Can you work these out from the model? Positions are in its coordinate system, mm. Face numbers are marked on the shaded views. A direction names the side the tool comes from. Give positions to 0.01 mm unless a question says otherwise; leave off trailing zeros. Loops run counter-clockwise (first coordinate to the right, second up) from the corner with the lowest first, then second, coordinate; pieces in that order, holes last. Notation, with made-up numbers: M -15,87.25 L 32,87.25 A38 ccw 32,126.25 Z; hole C -33,-28.75 d4. An arc over 180 degrees is marked long. Answer as a JSON object with one key per item and string values.
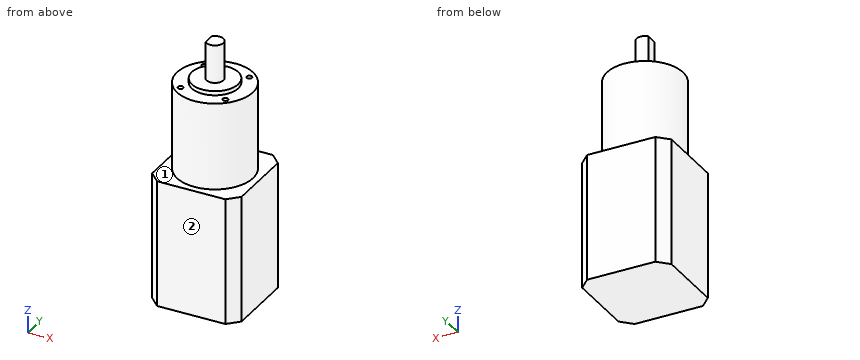
```python
from build123d import *

# Parameters (mm, degrees)
EXTRUDE_1_DEPTH        = 60
SKETCH_2_R             = 18
EXTRUDE_2_DEPTH        = 41.3
SKETCH_3_R             = 11
EXTRUDE_3_DEPTH        = 2
SKETCH_4_R             = 4
EXTRUDE_4_DEPTH        = 18
SKETCH_5_W             = 8.09428643
SKETCH_5_H             = 13.450799509
CUT_EXTRUDE_1_DEPTH    = 15
SKETCH_6_R             = 1
CUT_EXTRUDE_2_DEPTH    = 5
HOLE_WIZARD_M3_1_D     = 2.5
HOLE_WIZARD_M3_1_DEPTH = 7.5
HOLE_WIZARD_M3_1_TIP   = 0.751075774


with BuildPart() as part:
    # 草图1 → 凸台-拉伸1 (new body)
    with BuildSketch(Plane.XY):
        Polygon((-21.15, 16.15), (-16.15, 21.15), (16.15, 21.15), (21.15, 16.15), (21.15, -16.15), (16.15, -21.15), (-16.15, -21.15), (-21.15, -16.15), align=None)
    extrude(amount=EXTRUDE_1_DEPTH)

    # 草图2 → 凸台-拉伸2 (add)
    with BuildSketch(Plane.XY.offset(60)):
        Circle(SKETCH_2_R)
    extrude(amount=EXTRUDE_2_DEPTH)

    # 草图3 → 凸台-拉伸3 (add)
    with BuildSketch(Plane.XY.offset(101.3)):
        Circle(SKETCH_3_R)
    extrude(amount=EXTRUDE_3_DEPTH)

    # 草图4 → 凸台-拉伸4 (add)
    with BuildSketch(Plane.XY.offset(103.3)):
        Circle(SKETCH_4_R)
    extrude(amount=EXTRUDE_4_DEPTH)

    # 草图5 → 切除-拉伸1 (cut)
    with BuildSketch(Plane.XY.offset(121.3)):
        with Locations((-7.047143215, -1.347451383)):
            Rectangle(SKETCH_5_W, SKETCH_5_H)
    extrude(amount=-CUT_EXTRUDE_1_DEPTH, mode=Mode.SUBTRACT)

    # 草图6 → 切除-拉伸2 (cut)
    with BuildSketch(Plane.XY.offset(101.3)):
        with Locations((-10.606601718, 10.606601718)):
            Circle(SKETCH_6_R)
        with Locations((10.606601718, 10.606601718)):
            Circle(SKETCH_6_R)
        with Locations((-10.606601718, -10.606601718)):
            Circle(SKETCH_6_R)
        with Locations((10.606601718, -10.606601718)):
            Circle(SKETCH_6_R)
    extrude(amount=-CUT_EXTRUDE_2_DEPTH, mode=Mode.SUBTRACT)

    # M3 螺纹孔1
    with Locations(Plane.XY.offset(101.3)):
        with Locations((-10.606601718, 10.606601718), (10.606601718, 10.606601718), (-10.606601718, -10.606601718), (10.606601718, -10.606601718)):
            Hole(HOLE_WIZARD_M3_1_D / 2, depth=HOLE_WIZARD_M3_1_DEPTH)
            with Locations((0, 0, -(HOLE_WIZARD_M3_1_DEPTH + HOLE_WIZARD_M3_1_TIP / 2))):  # 118° drill point
                Cone(0, HOLE_WIZARD_M3_1_D / 2, HOLE_WIZARD_M3_1_TIP, mode=Mode.SUBTRACT)


solid = part.part
```
1) Suppose I cut it at D-D, the plane y = 14.5. Write out the boundary of the cut face in (x, z).
Answer list:
{"outline": "M -21.15,0 L 21.15,0 L 21.15,60 L 10.67,60 L 10.67,101.3 L -10.67,101.3 L -10.67,60 L -21.15,60 Z"}
2) Will these pins go through, and if not, where does the flat tip stop? pin 1 Ø8 at (y, z) = (-5.5, 67.5) entering from -X; pin 2 Ø21 at (x, y) = (-9, -6) entering from +Z; pin 3 Ø8 at (x, z) = (16, 88.5) entering from +Y; pin 4 Ø3 at (x, z) = (-1, 77.5) entering from +Y.
Answer list:
{"pin 1": "x = -17.94", "pin 2": "z = 121.3", "pin 3": "y = 13.42", "pin 4": "y = 18"}
3) Suppose I cut it at C-C, the plane z = 58.5. Write out the boundary of the cut face in (x, y), and give its area (3 significant figures).
Answer list:
{"outline": "M -21.15,-16.15 L -16.15,-21.15 L 16.15,-21.15 L 21.15,-16.15 L 21.15,16.15 L 16.15,21.15 L -16.15,21.15 L -21.15,16.15 Z", "area": "1,740 mm^2"}
4) For the marked faces 1 and 2, which set-ups out of +Z, -Z, +X, -X, +Y, -Y let a thin tool reach every point of the face, with its end or its side?
Answer list:
{"face 1": "+Z", "face 2": "+Z, -Z, +X, -X, -Y"}
5) Suppose I cut it at B-B, the plane x = 0. Write out the boundary of the cut face in (y, z).
Answer list:
{"outline": "M -21.15,0 L 21.15,0 L 21.15,60 L 18,60 L 18,101.3 L 11,101.3 L 11,103.3 L 4,103.3 L 4,121.3 L -4,121.3 L -4,103.3 L -11,103.3 L -11,101.3 L -18,101.3 L -18,60 L -21.15,60 Z"}
6) Please list where these lines run through material, in increasing order: line 1 along Z through (x, y) = (-4.5, 1.5); line 2 along Z through (x, y) = (-15, 15); line 3 along X through (y, z) = (10.5, 64). Write a range as from..to.
Answer list:
{"line 1": "0..103.3", "line 2": "0..60", "line 3": "-14.62..14.62"}
7) Suppose I cut it at A-A, the plane y = 0. Write out the boundary of the cut face in (x, z).
Answer list:
{"outline": "M -21.15,0 L 21.15,0 L 21.15,60 L 18,60 L 18,101.3 L 11,101.3 L 11,103.3 L 4,103.3 L 4,121.3 L -3,121.3 L -3,106.3 L -4,106.3 L -4,103.3 L -11,103.3 L -11,101.3 L -18,101.3 L -18,60 L -21.15,60 Z"}
